Design review of the part shown in the three views and the two pictorial views. Dimensions are in mm from the part's minimum x, y and z. Give positions to 0.01 mm unless a question says otherwise; leave off trailing zeros. Loops run counter-clockwise (first coordinate to the right, second up) from the corner with the lowest first, then second, coordinate; pieces in that order, holes last. Notation, with made-up numbers: (83, -14.75) -> (110, -14.75) arc R20 ccw to (110, 21.25) -> close; hole circle Ø11 at (-39, -18). An arc over 180 degrees is marked (long way). Answer as CSV lines item,"result".
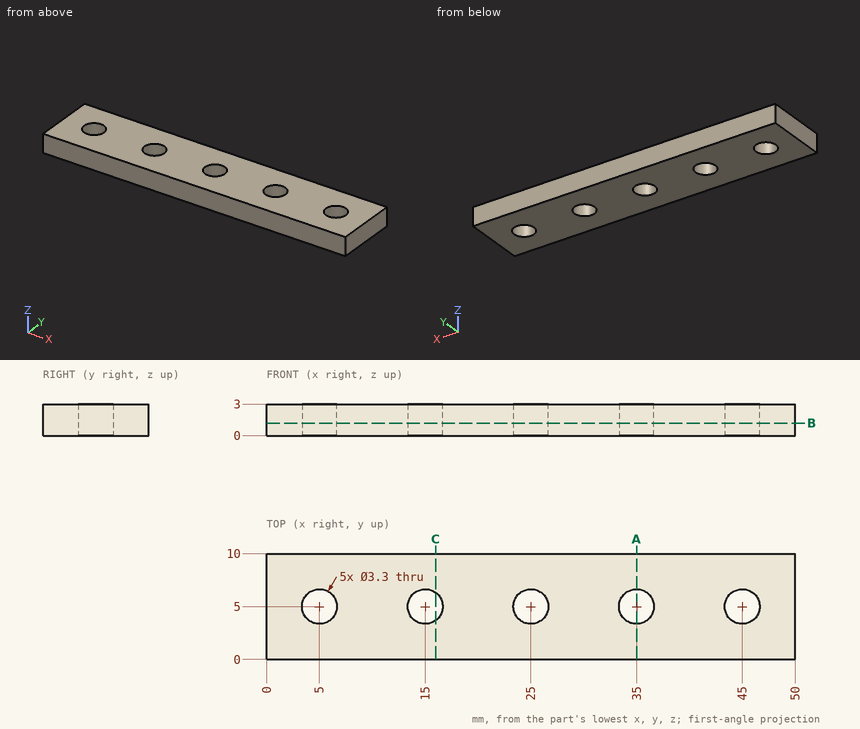
Q1. To check wall thickness, follow probe 1 along X at (y, z) = (5, 0.35); probe 2 along X at (y, z) = (3.5, 0.2); probe 3 along Y at (x, z) = (35, 1.3). State the ranges of each line that lie inside material, in increasing order. Write a range as from..to.
Filled sheet:
probe 1,"x = 0..3.35, 6.65..13.35, 16.65..23.35, 26.65..33.35, 36.65..43.35, 46.65..50"
probe 2,"x = 0..4.31, 5.69..14.31, 15.69..24.31, 25.69..34.31, 35.69..44.31, 45.69..50"
probe 3,"y = 0..3.35, 6.65..10"
Q2. We need section C-C, the plane x = 16. State the section outline as (y, z) points, and give its area (3 significant figures).
Filled sheet:
outline,"(0, 0) -> (3.69, 0) -> (3.69, 3) -> (0, 3) -> close; (6.31, 0) -> (10, 0) -> (10, 3) -> (6.31, 3) -> close"
area,"22.1 mm^2"
Q3. We need section B-B, the plane z = 1.2. State the section outline as (x, y) points, and give its area (3 significant figures).
Filled sheet:
outline,"(0, 0) -> (50, 0) -> (50, 10) -> (0, 10) -> close; hole circle Ø3.3 at (5, 5); hole circle Ø3.3 at (15, 5); hole circle Ø3.3 at (25, 5); hole circle Ø3.3 at (35, 5); hole circle Ø3.3 at (45, 5)"
area,"457 mm^2"
Q4. Clearance check with a flat-ended pin moving along its axis: pin 1 Ø2 at (x, y) = (45, 5) entering from -Z. State where the tip first meets the part, or that it passes through.
Filled sheet:
pin 1,"passes through"
Q5. We need section A-A, the plane x = 35. State the section outline as (y, z) points.
Filled sheet:
outline,"(0, 0) -> (3.35, 0) -> (3.35, 3) -> (0, 3) -> close; (6.65, 0) -> (10, 0) -> (10, 3) -> (6.65, 3) -> close"
